Verification items for the finished model (mm, model axes). A direction names the side the tool comes from. Coordinates: 2 decimals unless noted, no trailing zeros. Write each loop counter-clockwise with the first axis right and the second up, starting at its lowest first coordinate (ties: lowest second). Pieces come first, ordered by that corner, then holes.
```python
from build123d import *

# Parameters (mm, degrees)
SKETCH1_W           = 30
SKETCH1_H           = 40
BOSS_EXTRUDE1_DEPTH = 36
CUT_EXTRUDE1_START  = 14
CUT_EXTRUDE1_DEPTH  = 37.378214609
SKETCH4_R           = 2.35
CUT_EXTRUDE3_DEPTH  = 51.378214609
SKETCH5_R           = 6.5
CUT_EXTRUDE4_DEPTH  = 4
SKETCH12_R          = 5.25
SKETCH12_W          = 8
SKETCH12_H          = 20
CUT_EXTRUDE5_DEPTH  = 57.683017802
FILLET1_R           = 4


with BuildPart() as part:
    # Sketch1 → Boss-Extrude1 (new body)
    with BuildSketch(Plane(origin=(0, 0, 0), x_dir=(1, 0, 0), z_dir=(0, 1, 0))):
        with Locations((0, -11.889880952)):
            Rectangle(SKETCH1_W, SKETCH1_H)
    extrude(amount=BOSS_EXTRUDE1_DEPTH)

    # Sketch2 → Cut-Extrude1 (cut, through all)
    with BuildSketch(Plane.XZ.offset(-36).offset(CUT_EXTRUDE1_START)):
        Polygon((-11.25, 21.389880952), (-5.5, 21.389880952), (-5.5, 18.389880952), (5.5, 18.389880952), (5.5, 21.389880952), (11.25, 21.389880952), (11.25, 2.389880952), (5.5, 2.389880952), (5.5, 5.389880952), (-5.5, 5.389880952), (-5.5, 2.389880952), (-11.25, 2.389880952), align=None)
    extrude(amount=CUT_EXTRUDE1_DEPTH, mode=Mode.SUBTRACT)

    # Sketch4 → Cut-Extrude3 (cut, through all)
    with BuildSketch(Plane(origin=(0, 36, 0), x_dir=(1, 0, 0), z_dir=(0, 1, 0))):
        with Locations(Location((0, -11.889880952, 0), (0, 0, 270))):
            Circle(SKETCH4_R)
    extrude(amount=-CUT_EXTRUDE3_DEPTH, mode=Mode.SUBTRACT)

    # Sketch5 → Cut-Extrude4 (cut)
    with BuildSketch(Plane(origin=(0, 36, 0), x_dir=(1, 0, 0), z_dir=(0, 1, 0))):
        with Locations(Location((0, -11.889880952, 0), (0, 0, 270))):
            Circle(SKETCH5_R)
    extrude(amount=-CUT_EXTRUDE4_DEPTH, mode=Mode.SUBTRACT)

    # Sketch12 → Cut-Extrude5 (cut, through all)
    with BuildSketch(Plane.ZY.offset(15)):
        with Locations((0.889880952, 28)):
            Circle(SKETCH12_R)
        with Locations((22.889880952, 28)):
            Circle(SKETCH12_R)
        with Locations((-4.110119048, 10)):
            Rectangle(SKETCH12_W, SKETCH12_H)
        with Locations((27.889880952, 10)):
            Rectangle(SKETCH12_W, SKETCH12_H)
    extrude(amount=-CUT_EXTRUDE5_DEPTH, mode=Mode.SUBTRACT)

    # Fillet1
    # the kernel refuses this fillet: 4 mm, written as the material it adds along each edge
    with BuildSketch(Plane(origin=(-15, 20, -0.110119048), x_dir=(0, 0, -1), z_dir=(1, 0, 0)), Plane(origin=(-15, 20, 23.889880952), x_dir=(0, -1, 0), z_dir=(1, 0, 0))) as fillet1_piece_1:
        with BuildLine():
            CenterArc((FILLET1_R, -FILLET1_R), FILLET1_R, 90, 90)
            Line((0, -FILLET1_R), (0, 0))
            Line((0, 0), (FILLET1_R, 0))
        make_face()
    extrude(amount=30)
    # the kernel refuses this fillet: 4 mm, written as the material it takes off along each edge
    with BuildSketch(Plane(origin=(-25, 0, 23.889880952), x_dir=(0, 0, -1), z_dir=(1, 0, 0)), Plane(origin=(-25, 0, -0.110119048), x_dir=(0, 1, 0), z_dir=(1, 0, 0)), Plane(origin=(-25, 20, -8.110119048), x_dir=(0, 1, 0), z_dir=(1, 0, 0)), Plane(origin=(25, 36, 31.889880952), x_dir=(0, 0, -1), z_dir=(-1, 0, 0)), Plane(origin=(-25, 20, 31.889880952), x_dir=(0, 0, -1), z_dir=(1, 0, 0))) as fillet1_2_piece_1:
        with BuildLine():
            CenterArc((FILLET1_R, FILLET1_R), FILLET1_R, 180, 90)
            Line((0, FILLET1_R), (0, 0))
            Line((0, 0), (FILLET1_R, 0))
        make_face()
    extrude(amount=50, mode=Mode.SUBTRACT)
    with BuildSketch(Plane(origin=(-25, 36, -8.110119048), x_dir=(0, -1, 0), z_dir=(1, 0, 0))) as fillet1_2_piece_2:
        with BuildLine():
            CenterArc((FILLET1_R, -FILLET1_R), FILLET1_R, 90, 90)
            Line((0, -FILLET1_R), (0, 0))
            Line((0, 0), (FILLET1_R, 0))
        make_face()
    extrude(amount=50, mode=Mode.SUBTRACT)


solid = part.part
```
1. Draft check along Z on faces 4 (the flat face through (0, 10, -0.11)), 5 (the flat face through (0, 11, 18.39)), 6 (the flat face through (0, 0, 19)). Enter one of: pulls with the +Z half, pulls with the -Z half, needs draft (parallel to the pull), parting line crosses it, or undercut.
2. Material ranges on L1, parallel to Z at x = -3.5, y = 16; L2, parallel to X at y = 3, z = 16; L3, parallel to X at y = 12.5, z = 20.5, recorded low to high.
3. Gauge pin test, flat ends, axial feed: P1, Ø7.5, axis at x = 0, z = 11.89, coming from the +Y side; P2, Ø1.5, axis at x = -3, z = 16.5, coming from the -Y side; P3, Ø1.7, axis at x = 7.5, y = 11, coming from the -Z side. Record the tip position at first contact, or that the pin passes through.
4. Sectioned sample at C-C, the plane y = 8. Record the boundary of the cut face in (x, z).
5. Sectioned sample at D-D, the plane x = -7.75. Record the boundary of the cut face in (y, z), and give its area (3 significant figures).
6. Tool access check on faces 1 (the flat face through (0, 10, 23.89)), 2 (the flat face through (-5.5, 11, 4)), 3 (the cylindrical face through (-2.49, 34.028, 17.894)). Record the directions out of +Z, -Z, +X, -X, +Y, -Y that give a thin tool (end or side, any length) a straight path to the whole face; none if there is none.
7. Sectioned sample at B-B, the plane y = 28. Record the boundary of the cut face in (x, z), and give its area (3 significant figures).
8. Sectioned sample at A-A, the plane x = 0. Record the boundary of the cut face in (y, z).
Outcome:
1. face 4: pulls with the -Z half
1. face 5: undercut
1. face 6: needs draft
2. L1: z = -0.11 to 5.39, 18.39 to 23.89
2. L2: x = -15 to -11.25, 11.25 to 15
2. L3: x = -15 to -11.25, -5.5 to 5.5, 11.25 to 15
3. P1: stops at y = 32
3. P2: stops at y = 22
3. P3: stops at z = -0.11
4. outline: (-15, -0.11) - (15, -0.11) - (15, 23.89) - (-15, 23.89) - close; hole (-11.25, 2.39) - (-5.5, 2.39) - (-5.5, 5.39) - (5.5, 5.39) - (5.5, 2.39) - (11.25, 2.39) - (11.25, 21.39) - (5.5, 21.39) - (5.5, 18.39) - (-5.5, 18.39) - (-5.5, 21.39) - (-11.25, 21.39) - close
5. outline: (0.29, 2.39) arc R4 ccw to (4, -0.11) - (16, -0.11) arc R4 cw to (20, -4.11) arc R4 ccw to (24, -8.11) - (32, -8.11) arc R4 ccw to (36, -4.11) - (36, 27.89) arc R4 ccw to (32, 31.89) - (24, 31.89) arc R4 ccw to (20, 27.89) arc R4 cw to (16, 23.89) - (4, 23.89) arc R4 ccw to (0.29, 21.39) - (22, 21.39) - (22, 2.39) - close; hole circle Ø10.5 at (28, 0.89); hole circle Ø10.5 at (28, 22.89)
5. area: 515 mm2
6. face 1: +Z, +X, -X, -Y
6. face 2: -Y
6. face 3: +Y
7. outline: (-15, -8.11) - (15, -8.11) - (15, -4.36) - (-15, -4.36) - close; (-15, 6.14) - (15, 6.14) - (15, 17.64) - (-15, 17.64) - close; (-15, 28.14) - (15, 28.14) - (15, 31.89) - (-15, 31.89) - close; hole circle Ø4.7 at (0, 11.89)
7. area: 553 mm2
8. outline: (0, 3.89) arc R4 ccw to (4, -0.11) - (16, -0.11) arc R4 cw to (20, -4.11) arc R4 ccw to (24, -8.11) - (32, -8.11) arc R4 ccw to (36, -4.11) - (36, 5.39) - (32, 5.39) - (32, 9.54) - (22, 9.54) - (22, 5.39) - (0, 5.39) - close; (0, 18.39) - (22, 18.39) - (22, 14.24) - (32, 14.24) - (32, 18.39) - (36, 18.39) - (36, 27.89) arc R4 ccw to (32, 31.89) - (24, 31.89) arc R4 ccw to (20, 27.89) arc R4 cw to (16, 23.89) - (4, 23.89) arc R4 ccw to (0, 19.89) - close; hole circle Ø10.5 at (28, 0.89); hole circle Ø10.5 at (28, 22.89)
